For this review, use the dimensioned drawing (mm, ordinates from the lowest corner) and the shaded views. Give positions to 0.01 mm unless a question says otherwise; leave off trailing zeros. Write each loop counter-clockwise with the first axis right and the second up, starting at its lowest first coordinate (ties: lowest second). Pieces come first, ordered by that corner, then holes. Notation, with made-up numbers: M 40,79.25 L 64,79.25 A35 cw 64,112.25 Z; hole C 26.25,-19 d7. An arc over 180 degrees is marked long. One line per item, written item: value. Start each with the question number.
Item 1: Consider section C-C, the plane y = 1.75. Write out the cut boundary in (x, z).
Item 2: Clearance check with a flat-ended pin moving along its axis: pin 1 Ø3.5 at (x, z) = (22.18, 19) entering from +Y. State where the tip first meets the part, or that it passes through.
Item 3: To check wall thickness, follow probe 1 along X at (y, z) = (2.8, 79); probe 2 along Z at (x, y) = (131, 1.3). State the ranges of each line that lie inside material, in increasing order.
Item 4: Consider section B-B, the plane z = 113.5. Write out the cut boundary in (x, y).
Item 5: Consider section A-A, the plane x = 103. Write out the cut boundary in (y, z), and give its area (3 significant figures).
Item 6: Consider section D-D, the plane x = 131. Write out the cut boundary in (y, z).
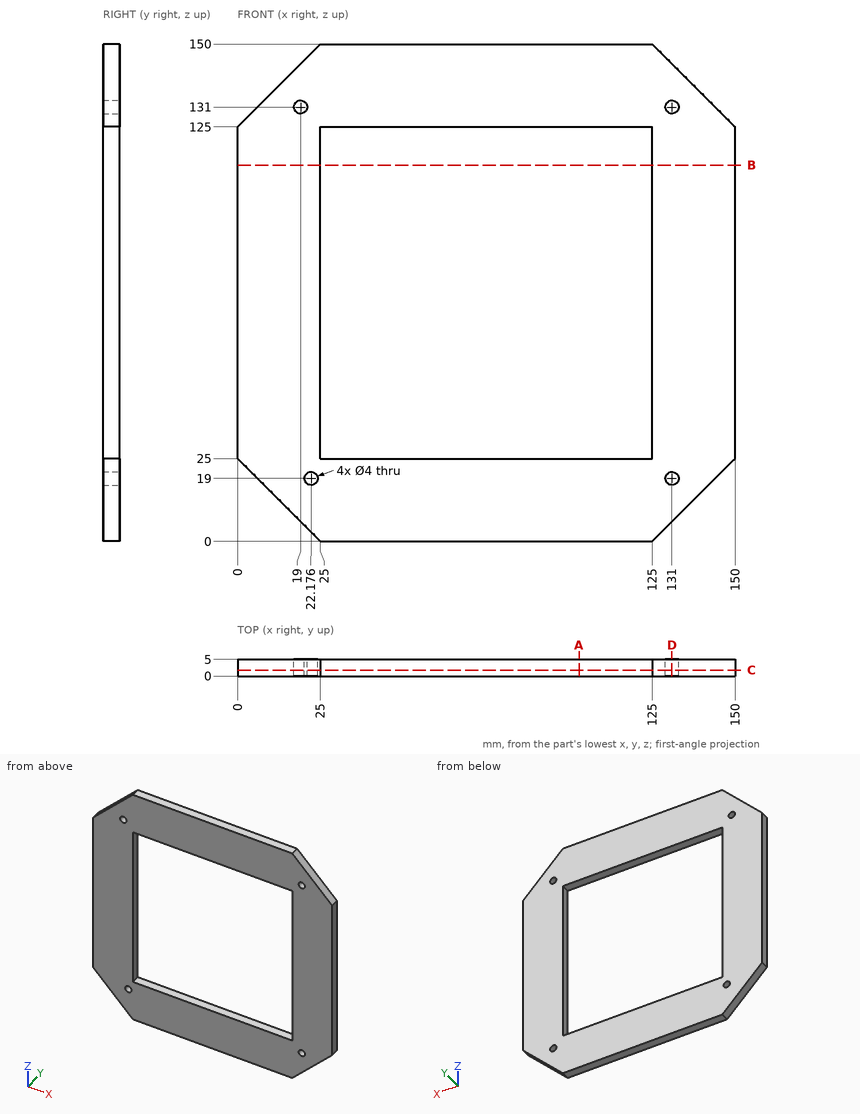
Model answer:
1. outline: M 0,25 L 25,0 L 125,0 L 150,25 L 150,125 L 125,150 L 25,150 L 0,125 Z; hole C 19,131 d4; hole C 22.18,19 d4; hole M 25,25 L 125,25 L 125,125 L 25,125 Z; hole C 131,19 d4; hole C 131,131 d4
2. pin 1: passes through
3. probe 1: x = 0 to 25, 125 to 150
3. probe 2: z = 6 to 17, 21 to 129, 133 to 144
4. outline: M 0,0 L 25,0 L 25,5 L 0,5 Z; M 125,0 L 150,0 L 150,5 L 125,5 Z
5. outline: M 0,0 L 5,0 L 5,25 L 0,25 Z; M 0,125 L 5,125 L 5,150 L 0,150 Z
5. area: 250 mm2
6. outline: M 0,6 L 5,6 L 5,17 L 0,17 Z; M 0,21 L 5,21 L 5,129 L 0,129 Z; M 0,133 L 5,133 L 5,144 L 0,144 Z
